Can you work these out from the drawing? Everything is in mm from the part's minimum corner. A direction names the side the tool comes from. Round coordinates to 2 decimals unless told otherwise and drop trailing zeros. Loops run counter-clockwise (first coordinate to the right, second up) from the corner with the lowest first, then second, coordinate; pieces in that order, holes last. Notation, with made-up numbers: (89, -16) -> (107, -16) arc R21 ccw to (107, 19) -> close; hole circle Ø5 at (45.5, 83.5). An arc over 180 degrees is marked (long way). Answer as a JSON object with one key per item and string values.
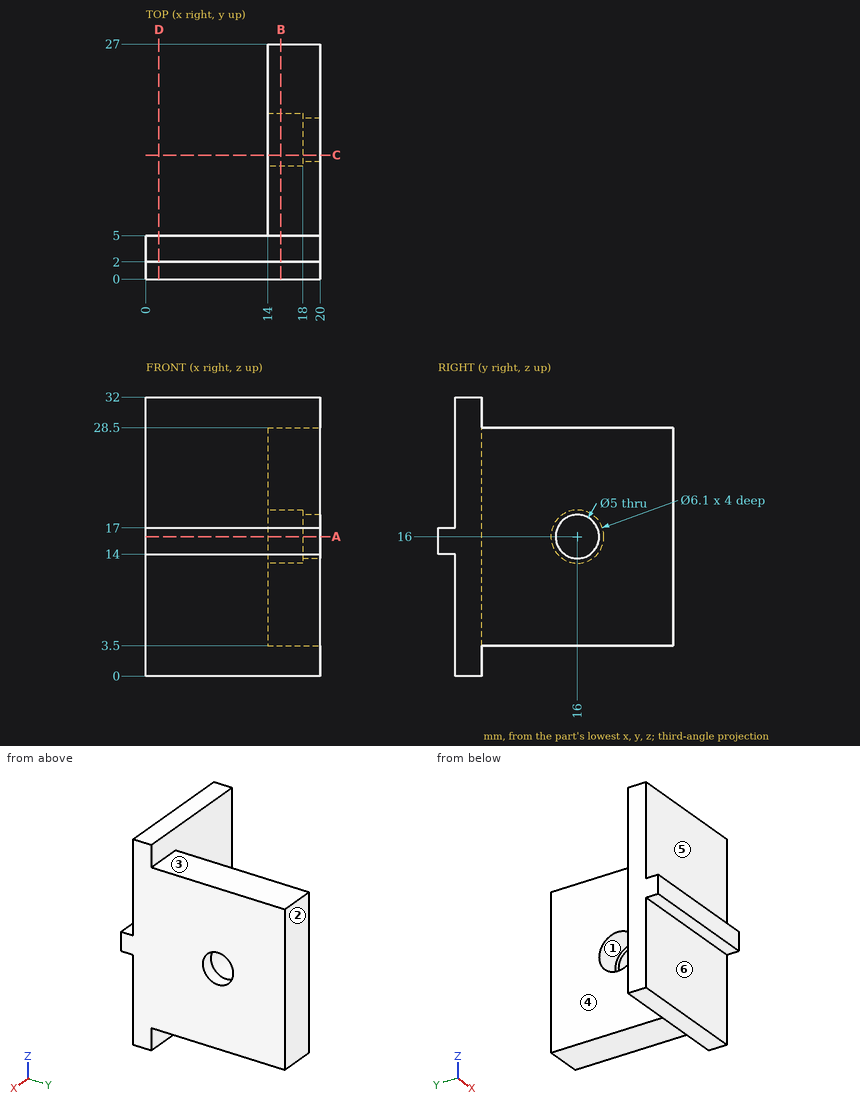
Q1. I want a section at A-A, the plane z = 16. Write out the boundary of the cut face in (x, y).
Determined:
{"outline": "(0, 0) -> (20, 0) -> (20, 13.5) -> (18, 13.5) -> (18, 12.95) -> (14, 12.95) -> (14, 5) -> (0, 5) -> close; (14, 19.05) -> (18, 19.05) -> (18, 18.5) -> (20, 18.5) -> (20, 27) -> (14, 27) -> close"}
Q2. I'm going to push flat-ended pins straight in: pin 1 (7 mm diameter, centred on y = 16, z = 16, fed in from -X); pin 2 (5 mm diameter, centred on x = 18, y = 15.5, fed in from +Z); pin 3 (1.6 mm diameter, centred on x = 12.5, y = 1, fed in from +Z); pin 4 (6 mm diameter, centred on x = 8, y = 3, fed in from -Z). Where does each tip first touch, or does it pass through?
Determined:
{"pin 1": "x = 14", "pin 2": "z = 28.5", "pin 3": "z = 17", "pin 4": "z = 0"}
Q3. On a 3-axis mill with a long thin cutter (end or side, diameter ignored), from which of +Z, -Z, +X, -X, +Y, -Y can I reach the whole of each face in a straight line? I mean the marked faces 4, 5 and 6. Say none if no direction works.
Determined:
{"face 4": "+Z, -Z, -X, +Y", "face 5": "+Z, +X, -X, -Y", "face 6": "-Z, +X, -X, -Y"}
Q4. I want a section at D-D, the plane x = 1.5. Write out the boundary of the cut face in (y, z), then the cut area to 3 significant figures.
Determined:
{"outline": "(0, 14) -> (2, 14) -> (2, 0) -> (5, 0) -> (5, 32) -> (2, 32) -> (2, 17) -> (0, 17) -> close", "area": "102 mm²"}
Q5. If I drill on L1, parallel to Z at x = 16.75, y = 16; L2, parallel to Z at x = 18.5, y = 7.25; L3, parallel to X at y = 24, z = 20, over which ranges is the centre line in solid material (lowest first)? Write a range as [from, to].
Determined:
{"L1": "[3.5, 12.95], [19.05, 28.5]", "L2": "[3.5, 28.5]", "L3": "[14, 20]"}
Q6. I want a section at C-C, the plane y = 14.25. Write out the boundary of the cut face in (x, z).
Determined:
{"outline": "(14, 3.5) -> (20, 3.5) -> (20, 14.21) -> (18, 14.21) -> (18, 13.5) -> (14, 13.5) -> close; (14, 18.5) -> (18, 18.5) -> (18, 17.79) -> (20, 17.79) -> (20, 28.5) -> (14, 28.5) -> close"}
Q7. I want a section at B-B, the plane x = 15.5. Write out the boundary of the cut face in (y, z), then the cut area to 3 significant figures.
Determined:
{"outline": "(0, 14) -> (2, 14) -> (2, 0) -> (5, 0) -> (5, 3.5) -> (27, 3.5) -> (27, 28.5) -> (5, 28.5) -> (5, 32) -> (2, 32) -> (2, 17) -> (0, 17) -> close; hole circle Ø6.1 at (16, 16)", "area": "623 mm²"}
Q8. We'd pull the mould along Z, two halves only. Please class the marked faces 1, 2 and 3: pulls with the +Z half, pulls with the -Z half, needs draft (parallel to the pull), parting line crosses it, or undercut.
Determined:
{"face 1": "undercut", "face 2": "needs draft", "face 3": "pulls with the +Z half"}
